Can you work these out from the model? Positions are in its coordinate system, mm. A direction names the side the tool comes from. Give positions to 0.01 mm unless a question says otherwise; leave off trailing zeros. Loops run counter-clockwise (first coordinate to the right, second up) from the corner with the lowest first, then second, coordinate; pieces in that order, holes last. Notation, with made-up numbers: (-16.75, 71.25) - (-9.75, 71.25) arc R8 ccw to (-9.75, 79.25) - close; hole circle Ø10 at (-9, -14.5). An arc over 180 degrees is marked (long way). Answer as a JSON object with one key per item and string values.
```python
from build123d import *

# Parameters (mm, degrees)
SKETCH1_W               = 115
SKETCH1_H               = 63.5
SKETCH1_R               = 1
PCB_DEPTH               = 1
CONNECTORS_DEPTH        = 3.5
CONNECTORS_DEPTH_BACK   = 0.5
SKETCH2_W               = 8
SKETCH2_H               = 12
SKETCH2_W_2             = 10
SKETCH2_H_2             = 10
SKETCH2_W_3             = 14
SKETCH2_H_3             = 6
SKETCH3_W               = 5
SKETCH3_H               = 26
DISPLAY_CONNECTOR_DEPTH = 1.5


with BuildPart() as part:
    # Sketch1 → PCB (new body)
    with BuildSketch(Plane(origin=(0, 0, 0), x_dir=(1, 0, 0), z_dir=(0, 1, 0))):
        Rectangle(SKETCH1_W, SKETCH1_H)
        with Locations(Location((-46.5, -25.25, 0), (0, 0, 270))):
            Circle(SKETCH1_R, mode=Mode.SUBTRACT)
        with Locations(Location((-36.5, 28.75, 0), (0, 0, 270))):
            Circle(SKETCH1_R, mode=Mode.SUBTRACT)
        with Locations(Location((41.5, 28.75, 0), (0, 0, 270))):
            Circle(SKETCH1_R, mode=Mode.SUBTRACT)
        with Locations(Location((41.5, -25.25, 0), (0, 0, 270))):
            Circle(SKETCH1_R, mode=Mode.SUBTRACT)
    extrude(amount=PCB_DEPTH)

    # Sketch2 → CONNECTORS (add, two sides: drawn at the far end of the back side and taken through both)
    with BuildSketch(Plane(origin=(0, 0, 0), x_dir=(1, 0, 0), z_dir=(0, 1, 0)).offset(-CONNECTORS_DEPTH_BACK)):
        with Locations((56, -21.75)):
            Rectangle(SKETCH2_W, SKETCH2_H)
        with Locations((55, -5.25)):
            Rectangle(SKETCH2_W_2, SKETCH2_H_2)
        with Locations((55, 11.75)):
            Rectangle(SKETCH2_W_2, SKETCH2_H_2)
        with Locations((53, 24.75)):
            Rectangle(SKETCH2_W_3, SKETCH2_H_3)
    extrude(amount=CONNECTORS_DEPTH + CONNECTORS_DEPTH_BACK)

    # Sketch3 → DISPLAY CONNECTOR (add)
    with BuildSketch(Plane(origin=(0, 1, 0), x_dir=(1, 0, 0), z_dir=(0, 1, 0))):
        with Locations((-53.5, -17.25)):
            Rectangle(SKETCH3_W, SKETCH3_H)
    extrude(amount=DISPLAY_CONNECTOR_DEPTH)


solid = part.part
```
1) Imagine slicing it at D-D on x = -39. Write out the boundary of the cut face in (y, z), and give its area (3 significant figures).
Check sheet entries:
{"outline": "(0, -31.75) - (1, -31.75) - (1, 31.75) - (0, 31.75) - close", "area": "63.5 mm2"}
2) Imagine slicing it at A-A on z = 22.5. Write out the boundary of the cut face in (x, y), and give its area (3 significant figures).
Check sheet entries:
{"outline": "(-57.5, 0) - (52, 0) - (52, -0.5) - (60, -0.5) - (60, 3.5) - (52, 3.5) - (52, 1) - (-51, 1) - (-51, 2.5) - (-56, 2.5) - (-56, 1) - (-57.5, 1) - close", "area": "149 mm2"}
3) If we mould it in two halves opening along Z, with no side actions, what happens to faces 1 (the flat face through (53, 2, -21.75)), 2 (the flat face through (60, 1, 22))? For each: released by +Z, released by -Z, zero draft, split by the parting line, or undercut.
Check sheet entries:
{"face 1": "undercut", "face 2": "zero draft"}
4) Imagine slicing it at C-C on z = -24. Write out the boundary of the cut face in (x, y), and give its area (4 significant figures).
Check sheet entries:
{"outline": "(-57.5, 0) - (46, 0) - (46, -0.5) - (60, -0.5) - (60, 3.5) - (46, 3.5) - (46, 1) - (-57.5, 1) - close", "area": "159.5 mm2"}
5) I need wall thicknesses on L1, parallel to X at y = 0.7, z = 25.25; L2, parallel to X at y = 0.6, z = -28.75; L3, parallel to Z at x = 54.5, y = 1.4. Which ranges of each line are inside material? Lowest first, please.
Check sheet entries:
{"L1": "-57.5 to -47.5, -45.5 to 40.5, 42.5 to 60", "L2": "-57.5 to -37.5, -35.5 to 40.5, 42.5 to 57.5", "L3": "-27.75 to -21.75, -16.75 to -6.75, 0.25 to 10.25, 15.75 to 27.75"}
6) I'm going to push flat-ended pins straight in: P1, Ø1.5, axis at x = -2, z = -2, coming from the -Y side; P2, Ø0.8, axis at y = 2, z = 15, coming from the +X side; P3, Ø0.8, axis at x = -54.5, y = 1.5, coming from the -Z side. Where does each tip first touch, or does it pass through?
Check sheet entries:
{"P1": "y = 0", "P2": "x = -51", "P3": "z = 4.25"}
7) Which directions (+Z, -Z, +X, -X, +Y, -Y) give clear straight access to the entire face, cutting with the end or side of a thin tool? Please do faces 3 (the flat face through (55, -0.5, 5)), 4 (the flat face through (50, 2, 5)), 5 (the flat face through (46, 2, -25)).
Check sheet entries:
{"face 3": "+Z, -Z, +X, -X, -Y", "face 4": "+Z, +Y", "face 5": "+Z, -Z, -X, +Y"}
8) Imagine slicing it at B-B on x = 48.5. Write out the boundary of the cut face in (y, z), and give its area (3 significant figures).
Check sheet entries:
{"outline": "(-0.5, -27.75) - (0, -27.75) - (0, -31.75) - (1, -31.75) - (1, -27.75) - (3.5, -27.75) - (3.5, -21.75) - (1, -21.75) - (1, 31.75) - (0, 31.75) - (0, -21.75) - (-0.5, -21.75) - close", "area": "81.5 mm2"}
